Can you work these out from the model? Positions are in its coordinate system, mm. A direction names the side the tool comes from. Round coordinates to 2 decimals unless told otherwise and drop trailing zeros. Order: outer loops, then holes, each group sorted by start corner. A loop starts at its lowest first (then second) coordinate and runs counter-clockwise, first axis right, second up.
from build123d import *

# Parameters (mm, degrees)
CROQUIS1_R                       = 6.125
SALIENTE_EXTRUIR1_DEPTH          = 9.53
BRIDA_DE_ARISTA1_STRIP_W         = 57.18
BRIDA_DE_ARISTA1_STRIP_H         = 9.53
BRIDA_DE_ARISTA1_STRIP_CUT_DEPTH = 85
BRIDA_DE_ARISTA1_DEPTH           = 85
REDONDEO3_R                      = 10
CHAFL_N1_START                   = 111.176977613
CHAFL_N1_OUTLINE_W               = 35
CHAFL_N1_OUTLINE_H               = 9.53
CHAFL_N1_DEPTH                   = 16.823022387
REDONDEO4_R                      = 20


with BuildPart() as part:
    # Croquis1 → Saliente-Extruir1 (new body)
    with BuildSketch(Plane.XY):
        with BuildLine():
            Line((-5, 12.5), (59.758688568, 12.5))
            ThreePointArc((59.758688568, 12.5), (63.068757982, 11.936283192), (66.005639043, 10.308688094))
            Line((66.005639043, 10.308688094), (70.527359279, 6.691311906))
            ThreePointArc((70.527359279, 6.691311906), (73.464240341, 5.063716808), (76.774309755, 4.5))
            Line((76.774309755, 4.5), (123.266499161, 4.5))
            ThreePointArc((123.266499161, 4.5), (125.848488059, 3.781744193), (127.688665549, 1.833333333))
            ThreePointArc((127.688665549, 1.833333333), (129.41356885, -2.692366017), (130, -7.5))
            Line((130, -7.5), (130, -37.5))
            Line((130, -37.5), (45, -37.5))
            Line((45, -37.5), (45, -22.5))
            Line((45, -22.5), (-5, -22.5))
            ThreePointArc((-5, -22.5), (-22.5, -5), (-5, 12.5))
        make_face()
        Circle(CROQUIS1_R, mode=Mode.SUBTRACT)
        with Locations((40, 0)):
            Circle(CROQUIS1_R, mode=Mode.SUBTRACT)
    extrude(amount=SALIENTE_EXTRUIR1_DEPTH)

    # Brida de arista1: sheet metal written as solids
    # Brida de arista1 strip (on a plane across the edge) → Brida de arista1 strip cut (cut)
    with BuildSketch(Plane(origin=(130, -37.5, 0), x_dir=(0, 1, 0), z_dir=(-1, 0, 0))):
        with Locations((-19.06, -4.765)):
            Rectangle(BRIDA_DE_ARISTA1_STRIP_W, BRIDA_DE_ARISTA1_STRIP_H)
    extrude(amount=BRIDA_DE_ARISTA1_STRIP_CUT_DEPTH, mode=Mode.SUBTRACT)

    # Brida de arista1 section (on a plane across the edge) → Brida de arista1 (add)
    with BuildSketch(Plane(origin=(130, -37.5, 0), x_dir=(0, 1, 0), z_dir=(-1, 0, 0))):
        with BuildLine():
            Line((-9.53, 9.53), (-9.53, 40.47))
            Line((-9.53, 40.47), (0, 40.47))
            Line((0, 40.47), (0, 9.53))
            ThreePointArc((0, 9.53), (2.791272375, 2.791272375), (9.53, 0))
            Line((9.53, 0), (9.53, -9.53))
            ThreePointArc((9.53, -9.53), (-3.947455249, -3.947455249), (-9.53, 9.53))
        make_face()
    extrude(amount=BRIDA_DE_ARISTA1_DEPTH)

    # Redondeo3
    redondeo3_edges = [part.edges().sort_by_distance(p)[0] for p in [
        (45, -22.5, 4.765),
        (45, -42.265, -40.47),
    ]]
    fillet(redondeo3_edges, radius=REDONDEO3_R)

    # Chaflán1: read off the stored shape, not the designer's step
    # Chaflán1 outline → Chaflán1 (cut)
    with BuildSketch(Plane(origin=(0, 0, 0), x_dir=(0.6246950475544231, 0, 0.7808688094430313), z_dir=(0.7808688094430313, 0, -0.6246950475544232)).offset(CHAFL_N1_START)):
        with Locations((53.5, 42.265)):
            Rectangle(CHAFL_N1_OUTLINE_W, CHAFL_N1_OUTLINE_H)
    extrude(amount=CHAFL_N1_DEPTH, mode=Mode.SUBTRACT)

    # Redondeo4
    redondeo4_edges = [part.edges().sort_by_distance(p)[0] for p in [
        (110, -42.265, -40.47),
        (130, -42.265, -15.47),
    ]]
    fillet(redondeo4_edges, radius=REDONDEO4_R)


solid = part.part
(1) I want a section at D-D, the plane x = 96. List the corners of the cut face in (y, z) for me, plus the area to 3 significant figures.
(2) I want a section at B-B, the plane x = 0. List the corners of the cut face in (y, z) for me (3 decimals).
(3) I want a section at A-A, the plane y = 0. List the corners of the cut face in (x, z) for me (1 decimal).
(4) I'm going to push flat-ended pins straight in: pin 1 Ø10.5 at (x, z) = (106, 5.5) entering from +Y; pin 2 Ø5 at (x, y) = (57.5, -14.5) entering from -Z; pin 3 Ø16 at (y, z) = (-43.5, -1.5) entering from -X; pin 4 Ø1 at (y, z) = (-1.5, -2) entering from -X. Where does each tip first touch, or does it pass through?
(5) If we mould it in two halves opening along X, with no side actions, what happens to faces 4 (the face through (42.15, -25.51, 4.27)), 5 (the face through (3.293, 5.165, 4.698)), 6 (the face through (27, 12.5, 5))? For each: pulls with the +X half, pulls with the -X half, needs draft (parallel to the pull), parting line crosses it, or undercut.
(6) Please list where these lines run through material, in increasing order: probe 1 along Y at (x, z) = (10, 3.5); probe 2 along Y at (x, z) = (0, 4.5) (3 decimals); probe 3 along Y at (x, z) = (40, 3.5) (3 decimals).
(7) On a 3-axis mill with a long thin cutter (end or side, diameter ignored), from which of +Z, -Z, +X, -X, +Y, -Y can I reach the whole of each face in a straight line? I mean faces 1 (the face through (88, -37.5, -25)), 2 (the face through (48.01, -42.2, -37.62)), 3 (the face through (100, 4.5, 5)). Say none if no direction works.
(8) I want a section at C-C, the plane z = 2. Give the number of separate pieces and of enclosed holes in the cut face, plus the area to 3 significant figures.
Ans:
1. outline: (-47.03, -40.47) - (-37.5, -40.47) - (-37.5, -9.53) arc R9.53 cw to (-27.97, 0) - (4.5, 0) - (4.5, 9.53) - (-27.97, 9.53) arc R19.06 ccw to (-47.03, -9.53) - close
1. area: 818 mm2
2. outline: (-22.5, 0) - (-6.125, 0) - (-6.125, 9.53) - (-22.5, 9.53) - close; (6.125, 0) - (12.5, 0) - (12.5, 9.53) - (6.125, 9.53) - close
3. outline: (-21.8, 0) - (-6.1, 0) - (-6.1, 9.5) - (-21.8, 9.5) - close; (6.1, 0) - (33.9, 0) - (33.9, 9.5) - (6.1, 9.5) - close; (46.1, 0) - (128.5, 0) - (128.5, 9.5) - (46.1, 9.5) - close
4. pin 1: stops at y = 4.5
4. pin 2: stops at z = 0
4. pin 3: stops at x = 45
4. pin 4: passes through
5. face 4: pulls with the -X half
5. face 5: undercut
5. face 6: needs draft
6. probe 1: y = -22.5 to 12.5
6. probe 2: y = -22.5 to -6.125, 6.125 to 12.5
6. probe 3: y = -23.84 to -6.125, 6.125 to 12.5
7. face 1: -Z, +X, -X, +Y
7. face 2: -Z, -X, +Y, -Y
7. face 3: +Z, -Z, +X, +Y
8. separate pieces: 1
8. enclosed holes: 2
8. area: 6,240 mm2
